```python
from build123d import *

# Parameters (mm, degrees)
F0_W      = 40
F0_H      = 68
F1_DEPTH  = 12
F2_W      = 5
F2_H      = 3
F3_DEPTH  = 59
F5_W      = 90
F5_H      = 68
F6_DEPTH  = 12
F7_W      = 3
F7_H      = 3
F8_DEPTH  = 200
F9_W      = 12
F9_H      = 68.2744067311
F9_H_2    = 68.7110256553
F10_DEPTH = 6


with BuildPart() as f1:
    # F0 (on Front) → F1 (new body)
    with BuildSketch(Plane.XZ):
        Rectangle(F0_W, F0_H)
    extrude(amount=F1_DEPTH)

    # F2 (on face) → F3 (cut)
    with BuildSketch(Plane.YZ.offset(20)):
        with Locations((-9.5, 22.5)):
            Rectangle(F2_W, F2_H)
    extrude(amount=-F3_DEPTH, mode=Mode.SUBTRACT)


with BuildPart() as f6:
    # F5 (on Front) → F6 (new body)
    with BuildSketch(Plane.XZ):
        Rectangle(F5_W, F5_H)
    extrude(amount=F6_DEPTH)

    # F7 (on face) → F8 (cut)
    with BuildSketch(Plane(origin=(-45, 0, 0), x_dir=(0, -1, 0), z_dir=(-1, 0, 0))):
        with Locations((10.5, 22.5)):
            Rectangle(F7_W, F7_H)
    extrude(amount=-F8_DEPTH, mode=Mode.SUBTRACT)

    # F9 (on face) → F10 (cut)
    with BuildSketch(Plane.XZ.offset(12)):
        with Locations((-39, 0.1372033656)):
            Rectangle(F9_W, F9_H)
        with Locations((39, 0.3555128276)):
            Rectangle(F9_W, F9_H_2)
    extrude(amount=-F10_DEPTH, mode=Mode.SUBTRACT)


solid = f6.part
```
Input: part model. Units: mm. Frame: model coordinates. A direction names the side the tool comes from. Round coordinates to 2 decimals unless told otherwise and drop trailing zeros. Loops run counter-clockwise (first coordinate to the right, second up) from the corner with the lowest first, then second, coordinate; pieces in that order, holes last. Notation, with made-up numbers: M 52,71 L 98,71 A34 cw 98,104 Z; hole C -17,-31.75 d7. An arc over 180 degrees is marked long. Answer in a Markdown table with one row per item. Add a question column.
1. Contact query for flat-ended pins moving along their axis: pin 1 (9.5 mm diameter, centred on x = 38.5, z = -17, fed in from -Y); pin 2 (3 mm diameter, centred on y = -8, z = 0.5, fed in from -X); pin 3 (1.8 mm diameter, centred on y = -8.5, z = -11, fed in from +X). Output: stop coordinate, or through.
2. Set-up query: faces 1 (the face through (39, -6, 0)), 2 (the face through (0, -10, 24)), 3 (the face through (-39, -6, 0)), 4 (the face through (-45, -3, 0)). Return all of +Z, -Z, +X, -X, +Y, -Y with unobstructed straight access to the full face (end or side cutting, diameter ignored); none if empty.
3. Section B-B (z = -8). Output: boundary loops of the cut face in (x, y), and give its area (3 significant figures).
4. Mould query, pull axis Z, two halves, no side actions, for faces 5 (the face through (-33, -9, 0)), 6 (the face through (-1, -6, -34)), 7 (the face through (0, -10, 21)), 8 (the face through (-1, -6, 34)). Classes: released by +Z, released by -Z, zero draft, split by the parting line, or undercut.
5. Ray query, probe 1 along Z at (x, y) = (25, -10); probe 2 along Y at (x, z) = (-40, -23.5); probe 3 along X at (y, z) = (-8.25, -27). Return the intervals inside material, ascending.
6. Section A-A (y = -10). Output: boundary loops of the cut face in (x, z), and give its area (3 significant figures).
Values follow:
| question | item | result |
|---|---|---|
| 1 | pin 1 | y = -6 |
| 1 | pin 2 | x = -33 |
| 1 | pin 3 | x = 33 |
| 2 | face 1 | +Z, -Z, +X, -Y |
| 2 | face 2 | +X, -X, -Y |
| 2 | face 3 | +Z, -Z, -X, -Y |
| 2 | face 4 | +Z, -Z, -X, +Y, -Y |
| 3 | outline | M -45,-6 L -33,-6 L -33,-12 L 33,-12 L 33,-6 L 45,-6 L 45,0 L -45,0 Z |
| 3 | area | 936 mm^2 |
| 4 | face 5 | zero draft |
| 4 | face 6 | released by -Z |
| 4 | face 7 | undercut |
| 4 | face 8 | released by +Z |
| 5 | probe 1 | -34 to 21, 24 to 34 |
| 5 | probe 2 | -6 to 0 |
| 5 | probe 3 | -33 to 33 |
| 6 | outline | M -33,-34 L 33,-34 L 33,21 L -33,21 Z; M -33,24 L 33,24 L 33,34 L -33,34 Z |
| 6 | area | 4,290 mm^2 |
